from build123d import *

# Parameters (mm, degrees)
SKETCH1_W                     = 100
SKETCH1_H                     = 30
SKETCH1_R                     = 1.625
BOSS_EXTRUDE1_DEPTH           = 10
FILLET1_R                     = 15
CBORE_FOR_M3_SHCS_D           = 3.4
CBORE_FOR_M3_SHCS_DEPTH       = 23
CBORE_FOR_M3_SHCS_CBORE_D     = 6.5
CBORE_FOR_M3_SHCS_CBORE_DEPTH = 3
CBORE_FOR_M3_SHCS_TIP         = 1.021463052


with BuildPart() as part:
    # Sketch1 → Boss-Extrude1 (new body)
    with BuildSketch(Plane(origin=(0, 0, 0), x_dir=(0, 0, -1), z_dir=(1, 0, 0))):
        Rectangle(SKETCH1_W, SKETCH1_H)
        with Locations((-30, 5)):
            Circle(SKETCH1_R, mode=Mode.SUBTRACT)
    extrude(amount=BOSS_EXTRUDE1_DEPTH)

    # Fillet1
    fillet1_edges = [part.edges().sort_by_distance(p)[0] for p in [
        (5, -15, 50),
    ]]
    fillet(fillet1_edges, radius=FILLET1_R)

    # CBORE for M3 SHCS
    with Locations(Plane(origin=(-726.293536786, 25, -1323.282701689), x_dir=(1, 0, 0), z_dir=(0, 1, 0))):
        with Locations((731.293536786, -1281.282701689), (731.293536786, -1359.282701689), (621.293536786, -1281.282701689), (621.293536786, -1365.282701689), (621.293536786, -1323.282701689), (731.293536786, -1320.282701689)):
            CounterBoreHole(CBORE_FOR_M3_SHCS_D / 2, CBORE_FOR_M3_SHCS_CBORE_D / 2, CBORE_FOR_M3_SHCS_CBORE_DEPTH, depth=CBORE_FOR_M3_SHCS_DEPTH)
            with Locations((0, 0, -(CBORE_FOR_M3_SHCS_DEPTH + CBORE_FOR_M3_SHCS_TIP / 2))):  # 118° drill point
                Cone(0, CBORE_FOR_M3_SHCS_D / 2, CBORE_FOR_M3_SHCS_TIP, mode=Mode.SUBTRACT)


solid = part.part
Model file for the job. Use its own axes, mm. A direction names the side the tool comes from. Give positions to 0.01 mm unless a question says otherwise; leave off trailing zeros. Loops run counter-clockwise (first coordinate to the right, second up) from the corner with the lowest first, then second, coordinate; pieces in that order, holes last.
Item 1: Slice it at C-C (x = 2). Write the cut outline in (y, z) (3 decimals).
Check values:
outline: (-15, -50) - (15, -50) - (15, 50) - (0, 50) arc R15 ccw to (-15, 35) - close; hole circle Ø3.25 at (5, 30)
Item 2: Slice it at A-A (y = 5). Write the cut outline in (x, z) (3 decimals), plus the area to 3 significant figures.
Check values:
outline: (0, -50) - (10, -50) - (10, 28.375) - (0, 28.375) - close; (0, 31.625) - (10, 31.625) - (10, 50) - (0, 50) - close; hole circle Ø3.4 at (5, -42); hole circle Ø3.4 at (5, -3); hole circle Ø3.4 at (5, 36)
area: 940 mm2
Item 3: Mould opens along X. For faces 3 (the face through (0, 0, 1)), 4 (the face through (5.07, -10.49, 45.72)), 5 (the face through (5.273, 1.156, -2.887)), 6 (the face through (4.962, 1.156, -42.293)) say: +X half, -X half, draft (parallel to the pull), parting line (faces both ways), or undercut.
Check values:
face 3: -X half
face 4: draft
face 5: undercut
face 6: undercut
Item 4: Which spindle directions (+Z, -Z, +X, -X, +Y, -Y) get a long thin tool onto all of the face, cutting with end or side? Do faces 1 (the face through (5, -15, -7)), 2 (the face through (5.37, 8.41, 37.66)). Say none if no direction does.
Check values:
face 1: +Z, -Z, +X, -X, -Y
face 2: +Y
Item 5: Drop flat-ended pins along their axis: P1, Ø5, axis at x = 5, y = -12, coming from the +Z side; P2, Ø2, axis at x = 5, z = -42, coming from the +Y side. Give the stop position or say it passes through.
Check values:
P1: stops at z = 46.61
P2: stops at y = 1.58
Item 6: Drill centre lines: line 1 along Z through (x, y) = (5, 7.5); line 2 along X through (y, z) = (5.5, -42); line 3 along Z through (x, y) = (6.5, 12.5). Where is each one in solid material? Low to high.
Check values:
line 1: z = -50 to -43.7, -40.3 to -4.7, -1.3 to 34.3, 37.7 to 50
line 2: x = 0 to 3.3, 6.7 to 10
line 3: z = -50 to -42.8, -41.2 to -3.8, -2.2 to 35.2, 36.8 to 50
Item 7: Slice it at B-B (z = 30). Write the cut outline in (x, y) (3 decimals).
Check values:
outline: (0, -15) - (10, -15) - (10, 3.375) - (0, 3.375) - close; (0, 6.625) - (10, 6.625) - (10, 15) - (0, 15) - close
